```python
from build123d import *

# Parameters (mm, degrees)
BOSS_EXTRUDE1_DEPTH = 5
BOSS_EXTRUDE2_START = -5
SKETCH6_W           = 3
SKETCH6_H           = 3
SKETCH6_H_2         = 1.5
SKETCH6_W_2         = 10
BOSS_EXTRUDE2_DEPTH = 60
SKETCH7_W           = 46
SKETCH7_H           = 4.5
BOSS_EXTRUDE3_DEPTH = 3
SKETCH8_W           = 50
SKETCH8_H           = 70
CUT_EXTRUDE2_DEPTH  = 1
SKETCH9_R           = 1
BOSS_EXTRUDE4_DEPTH = 1
CUT_EXTRUDE3_REACH  = 52.551
SKETCH10_W          = 13.006782721
SKETCH10_H          = 17.639239295


with BuildPart() as part:
    # Sketch4 → Boss-Extrude1 (new body)
    with BuildSketch(Plane(origin=(0, 0, 0), x_dir=(0, 1, 0), z_dir=(0, 0, 1))):
        Polygon((-39.75, -29.75), (-14.905444566, -29.75), (-16.637495374, -26.75), (0.24999995, -26.75), (17.137495374, -26.75), (15.405444566, -29.75), (39.75, -29.75), (39.75, -10), (36.75, -10), (36.75, 10), (39.75, 10), (39.75, 29.75), (15.405444566, 29.75), (17.137495374, 26.75), (0.250000065, 26.75), (-16.637495374, 26.75), (-14.905444566, 29.75), (-39.75, 29.75), (-39.75, 10), (-36.75, 10), (-36.75, -10), (-39.75, -10), align=None)
    extrude(amount=BOSS_EXTRUDE1_DEPTH)

    # Sketch6 → Boss-Extrude2 (add)
    with BuildSketch(Plane.XZ.offset(36.75).offset(BOSS_EXTRUDE2_START)):
        with Locations((-21.528635138, 6.5)):
            Rectangle(SKETCH6_W, SKETCH6_H)
        with Locations((-21.528635138, 8.75)):
            Rectangle(SKETCH6_W, SKETCH6_H_2)
        with Locations((-15.028635138, 8.75)):
            Rectangle(SKETCH6_W_2, SKETCH6_H_2)
        with Locations((21.471364862, 6.5)):
            Rectangle(SKETCH6_W, SKETCH6_H)
        with Locations((21.471364862, 8.75)):
            Rectangle(SKETCH6_W, SKETCH6_H_2)
        with Locations((14.971364862, 8.75)):
            Rectangle(SKETCH6_W_2, SKETCH6_H_2)
    extrude(amount=-BOSS_EXTRUDE2_DEPTH)

    # Sketch7 → Boss-Extrude3 (add)
    with BuildSketch(Plane(origin=(0, 28.25, 0), x_dir=(-1, 0, 0), z_dir=(0, 1, 0))):
        with Locations((0.028635138, 7.25)):
            Rectangle(SKETCH7_W, SKETCH7_H)
    extrude(amount=BOSS_EXTRUDE3_DEPTH)

    # Sketch8 → Cut-Extrude2 (cut)
    with BuildSketch(Plane(origin=(0, 0, 0), x_dir=(1, 0, 0), z_dir=(0, 0, -1))):
        Rectangle(SKETCH8_W, SKETCH8_H)
    extrude(amount=-CUT_EXTRUDE2_DEPTH, mode=Mode.SUBTRACT)

    # Sketch9 → Boss-Extrude4 (add)
    # profile 1 of 14: a face of its own
    with BuildSketch(Plane(origin=(0, 0, 1), x_dir=(1, 0, 0), z_dir=(0, 0, -1))):
        with Locations((-12.786487011, -17.078606255)):
            Circle(SKETCH9_R)
    # profile 2 of 14: a face of its own
    with BuildSketch(Plane(origin=(0, 0, 1), x_dir=(1, 0, 0), z_dir=(0, 0, -1))):
        with Locations((-6.463434267, -17.078606255)):
            Circle(SKETCH9_R)
    # profile 3 of 14: a face of its own
    with BuildSketch(Plane(origin=(0, 0, 1), x_dir=(1, 0, 0), z_dir=(0, 0, -1))):
        with Locations((0, -17.078606255)):
            Circle(SKETCH9_R)
    # profile 4 of 14: a face of its own
    with BuildSketch(Plane(origin=(0, 0, 1), x_dir=(1, 0, 0), z_dir=(0, 0, -1))):
        with Locations((0, -14.125611289)):
            Circle(SKETCH9_R)
    # profile 5 of 14: a face of its own
    with BuildSketch(Plane(origin=(0, 0, 1), x_dir=(1, 0, 0), z_dir=(0, 0, -1))):
        with Locations((2.94008007, -14.125611289)):
            Circle(SKETCH9_R)
    # profile 6 of 14: a face of its own
    with BuildSketch(Plane(origin=(0, 0, 1), x_dir=(1, 0, 0), z_dir=(0, 0, -1))):
        with Locations((2.94008007, -11.346566296)):
            Circle(SKETCH9_R)
    # profile 7 of 14: a face of its own
    with BuildSketch(Plane(origin=(0, 0, 1), x_dir=(1, 0, 0), z_dir=(0, 0, -1))):
        with Locations((6.560973521, -11.346566296)):
            Circle(SKETCH9_R)
    # profile 8 of 14: a face of its own
    with BuildSketch(Plane(origin=(0, 0, 1), x_dir=(1, 0, 0), z_dir=(0, 0, -1))):
        with Locations((12.343594407, -11.346566296)):
            Circle(SKETCH9_R)
    # profile 9 of 14: a face of its own
    with BuildSketch(Plane(origin=(0, 0, 1), x_dir=(1, 0, 0), z_dir=(0, 0, -1))):
        with Locations((12.343594407, -14.125611289)):
            Circle(SKETCH9_R)
    # profile 10 of 14: a face of its own
    with BuildSketch(Plane(origin=(0, 0, 1), x_dir=(1, 0, 0), z_dir=(0, 0, -1))):
        with Locations((12.343594407, -17.078606255)):
            Circle(SKETCH9_R)
    # profile 11 of 14: a face of its own
    with BuildSketch(Plane(origin=(0, 0, 1), x_dir=(1, 0, 0), z_dir=(0, 0, -1))):
        with Locations((15.424056, -11.346566296)):
            Circle(SKETCH9_R)
    # profile 12 of 14: a face of its own
    with BuildSketch(Plane(origin=(0, 0, 1), x_dir=(1, 0, 0), z_dir=(0, 0, -1))):
        Polygon((-6.303627236, 4.647475362), (-9.872238462, 4.647475362), (-9.872238462, -6.382777516), (-11.332124872, -6.382777516), (-11.332124872, 4.647475362), (-14.900736097, 4.647475362), (-14.900736097, 5.945152171), (-6.303627236, 5.945152171), align=None)
    # profile 13 of 14: a face of its own
    with BuildSketch(Plane(origin=(0, 0, 1), x_dir=(1, 0, 0), z_dir=(0, 0, -1))):
        Polygon((5.213254446, -6.382777516), (3.606365584, -6.382777516), (2.30615425, -2.976375892), (-2.985933988, -2.976375892), (-4.199971471, -6.382777516), (-5.816998433, -6.382777516), (-1.062229499, 5.945152171), (0.440743837, 5.945152171), align=None)
        with BuildLine():
            Line((1.829663547, -1.678699083), (-0.132058817, 3.65647608))
            add(Edge.make_bspline(
                [(-0.132058817, 3.65647608), (-0.147664764, 3.706203134), (-0.182599633, 3.817520196), (-0.230569306, 4.004992715), (-0.27451989, 4.232251444), (-0.303796625, 4.396518738), (-0.319613669, 4.485265761)],
                knots=[0, 0, 0, 0, 0.735233958, 1.645866306, 2.728156085, 4, 4, 4, 4], degree=3))
            Line((-0.319613669, 4.485265761), (-0.352562494, 4.485265761))
            add(Edge.make_bspline(
                [(-0.352562494, 4.485265761), (-0.367323874, 4.402388942), (-0.395422699, 4.244629907), (-0.442062801, 4.022554742), (-0.494871195, 3.828782863), (-0.536126975, 3.711193738), (-0.555324495, 3.65647608)],
                knots=[0, 0, 0, 0, 1.1821815, 2.250325448, 3.185825268, 4, 4, 4, 4], degree=3))
            Line((-0.555324495, 3.65647608), (-2.506908759, -1.678699083))
            Line((-2.506908759, -1.678699083), (1.829663547, -1.678699083))
        make_face(mode=Mode.SUBTRACT)
    # profile 14 of 14: a face of its own
    with BuildSketch(Plane(origin=(0, 0, 1), x_dir=(1, 0, 0), z_dir=(0, 0, -1))):
        with BuildLine():
            Line((8.457446469, -1.678699083), (8.457446469, -6.382777516))
            Line((8.457446469, -6.382777516), (6.997560058, -6.382777516))
            Line((6.997560058, -6.382777516), (6.997560058, 5.945152171))
            Line((6.997560058, 5.945152171), (10.350736657, 5.945152171))
            add(Edge.make_bspline(
                [(10.350736657, 5.945152171), (10.509695311, 5.94250725), (10.818166439, 5.937374583), (11.266927294, 5.88984235), (11.688470568, 5.818158675), (12.083717966, 5.715231867), (12.449844904, 5.577532383), (12.788978426, 5.411630082), (13.10398336, 5.220680323), (13.384579674, 4.991925283), (13.640330715, 4.742713756), (13.858595137, 4.463555677), (14.046290599, 4.161729634), (14.198048848, 3.833912071), (14.314343043, 3.48152593), (14.397958134, 3.105462584), (14.449017319, 2.704893846), (14.455752673, 2.42907422), (14.459201711, 2.28783257)],
                knots=[0, 0, 0, 0, 1.220578922, 2.368624473, 3.462135539, 4.502544785, 5.500522599, 6.461134096, 7.399369976, 8.322607956, 9.235733545, 10.136695962, 11.037097352, 11.960312526, 12.90425338, 13.881897398, 14.915362519, 16, 16, 16, 16], degree=3))
            add(Edge.make_bspline(
                [(14.459201711, 2.28783257), (14.456125133, 2.145713753), (14.450093475, 1.867088625), (14.392842954, 1.458577322), (14.298798135, 1.070067677), (14.170811012, 0.698864827), (13.997972005, 0.351851734), (13.795716853, 0.020347803), (13.548830266, -0.286010644), (13.271970609, -0.574267746), (12.963200376, -0.836054299), (12.624253148, -1.061978102), (12.259784751, -1.253070736), (11.868668942, -1.407989064), (11.451812999, -1.528768286), (11.009560292, -1.618354116), (10.541130741, -1.668202008), (10.220744681, -1.675144873), (10.056731755, -1.678699083)],
                knots=[0, 0, 0, 0, 1.022395889, 2.004415688, 2.961535425, 3.896140743, 4.82343876, 5.746400737, 6.685563929, 7.648805907, 8.619636875, 9.592693104, 10.574524643, 11.576040996, 12.61506259, 13.694246144, 14.819632053, 16, 16, 16, 16], degree=3))
            Line((10.056731755, -1.678699083), (8.457446469, -1.678699083))
        make_face()
        with BuildLine():
            Line((8.457446469, 4.647475362), (8.457446469, -0.381022274))
            Line((8.457446469, -0.381022274), (9.957885279, -0.381022274))
            add(Edge.make_bspline(
                [(9.957885279, -0.381022274), (10.077940481, -0.379452684), (10.31093283, -0.376406565), (10.649599833, -0.342109598), (10.966509261, -0.289852539), (11.262229227, -0.217435817), (11.534525044, -0.120826947), (11.784771245, -0.00343225), (12.015027367, 0.132656375), (12.220130693, 0.293746461), (12.40507983, 0.471885839), (12.564099334, 0.670006443), (12.701263006, 0.885087886), (12.808528198, 1.119672064), (12.896289259, 1.369569482), (12.956358781, 1.637465518), (12.991871549, 1.922744559), (12.996789996, 2.118759427), (12.999315301, 2.219400395)],
                knots=[0, 0, 0, 0, 1.265277681, 2.455537233, 3.584498775, 4.649494157, 5.660845971, 6.625094694, 7.559934571, 8.473920379, 9.368340756, 10.261385271, 11.146040016, 12.050559185, 12.974472874, 13.933813817, 14.939146914, 16, 16, 16, 16], degree=3))
            add(Edge.make_bspline(
                [(12.999315301, 2.219400395), (12.997979793, 2.317539924), (12.995379811, 2.508599083), (12.957720492, 2.784773853), (12.904092134, 3.042639571), (12.823919422, 3.279856734), (12.726105371, 3.500854512), (12.600929429, 3.700909707), (12.454878872, 3.883183964), (12.286699993, 4.047522092), (12.093084536, 4.187745781), (11.87946034, 4.311880083), (11.642587123, 4.414603882), (11.384078714, 4.500966841), (11.102977848, 4.565807264), (10.800766648, 4.614221035), (10.475423413, 4.641369896), (10.251093913, 4.6453968), (10.13530203, 4.647475362)],
                knots=[0, 0, 0, 0, 1.094831488, 2.131430464, 3.106461648, 4.031144782, 4.921863596, 5.798739979, 6.657572552, 7.524756014, 8.415225068, 9.319623649, 10.278320726, 11.292489325, 12.358664814, 13.495361146, 14.707183632, 16, 16, 16, 16], degree=3))
            Line((10.13530203, 4.647475362), (8.457446469, 4.647475362))
        make_face(mode=Mode.SUBTRACT)
    extrude(amount=BOSS_EXTRUDE4_DEPTH)

    # Cut-Extrude3: up to this face of the body (flat: up to its plane)
    cut_extrude3_end = Plane(part.part.faces().sort_by_distance((0.003637838, -0.898870224, 5))[0])
    # Sketch10 → Cut-Extrude3 (cut, up to the picked face)
    with BuildSketch(Plane.XY.offset(9.5), mode=Mode.PRIVATE) as cut_extrude3_sk1:
        with Locations((-16.525243778, -22.930380353)):
            Rectangle(SKETCH10_W, SKETCH10_H)
    cut_extrude3_tool1 = split(extrude(cut_extrude3_sk1.sketch, amount=-CUT_EXTRUDE3_REACH, mode=Mode.PRIVATE), bisect_by=cut_extrude3_end, keep=Keep.BOTH, mode=Mode.PRIVATE)
    add(cut_extrude3_tool1.solids().sort_by(Axis((-16.525244, -22.93038, 9.5), (0, 0, -1)))[0], mode=Mode.SUBTRACT)


solid = part.part
```
Source: CAD feature listing. Evaluate the final solid. Frame: model axes, mm. A direction names the side the tool comes from. Give positions to 0.01 mm unless a question says otherwise; leave off trailing zeros. Write each loop counter-clockwise with the first axis right and the second up, starting at its lowest first coordinate (ties: lowest second). Pieces come first, ordered by that corner, then holes. Notation, with made-up numbers: (77, 48) - (106, 48) arc R12 ccw to (106, 66) - close; hole circle Ø8 at (20, -18). An arc over 180 degrees is marked (long way). One line per item, written item: value. Start each with the question number.
Q1. Section query B-B, the plane y = -18.5. Return the cut outline in (x, z), then the cut area to 3 significant figures.
Q2. First-contact query: pin 1 Ø3.5 at (y, z) = (-10.5, 7) entering from +X; pin 2 Ø3 at (x, z) = (-13.5, 8.5) entering from -Y; pin 3 Ø0.8 at (y, z) = (-2, 0.5) entering from +X. Flat tips, straight axial feed; report the tip coordinate or a pass-through.
Q3. Section query A-A, the plane y = 19.5. Return the cut outline in (x, z).
Q4. Draft query along Y for faces 1 (the face through (2.794, 0.133, 0.507)), 2 (the face through (12, 17, 0)), 3 (the face through (0, 31.25, 7)). Return one class per face: +Y half, -Y half, draft (parallel to the pull), parting line (faces both ways), or undercut.
Q5. Material intervals for probe 1 along Z at (x, y) = (-13, 7); probe 2 along X at (y, z) = (16, 6.5); probe 3 along X at (y, z) = (31, 5.25), sorted ascending. Write a range as from..to.
Q6. Section query C-C, the plane y = 34. Return the cut outline in (x, z).
Q7. Set-up query: faces 4 (the face through (10, -38, 2)), 5 (the face through (22.971, -1, 7)), 6 (the face through (-20.029, 7, 6)), 7 (the face through (-1.517, -1.026, 0.507)). Return all of +Z, -Z, +X, -X, +Y, -Y with unobstructed straight access to the full face (end or side cutting, diameter ignored); none if empty.
Answer:
1. outline: (-29.75, 0) - (-25, 0) - (-25, 1) - (25, 1) - (25, 0) - (29.75, 0) - (29.75, 5) - (22.97, 5) - (22.97, 9.5) - (9.97, 9.5) - (9.97, 8) - (19.97, 8) - (19.97, 5) - (-29.75, 5) - close
1. area: 276 mm2
2. pin 1: stops at x = 22.97
2. pin 2: stops at y = -14.11
2. pin 3: stops at x = 26.75
3. outline: (-29.75, 0) - (-25, 0) - (-25, 1) - (25, 1) - (25, 0) - (29.75, 0) - (29.75, 5) - (22.97, 5) - (22.97, 9.5) - (9.97, 9.5) - (9.97, 8) - (19.97, 8) - (19.97, 5) - (-20.03, 5) - (-20.03, 8) - (-10.03, 8) - (-10.03, 9.5) - (-23.03, 9.5) - (-23.03, 5) - (-29.75, 5) - close
4. face 1: undercut
4. face 2: draft
4. face 3: +Y half
5. probe 1: z = 1..5, 8..9.5
5. probe 2: x = -23.03..-20.03, 19.97..22.97
5. probe 3: x = -23.03..22.97
6. outline: (-29.75, 0) - (-25, 0) - (-25, 1) - (25, 1) - (25, 0) - (29.75, 0) - (29.75, 5) - (-29.75, 5) - close
7. face 4: +Z, -Z, -Y
7. face 5: +Z, +X, +Y, -Y
7. face 6: -Y
7. face 7: -Z
